Verification items for the finished model (mm, model axes). Give positions to 0.01 mm unless a question says otherwise; leave off trailing zeros. Loops run counter-clockwise (first coordinate to the right, second up) from the corner with the lowest first, then second, coordinate; pieces in that order, holes last. Notation, with made-up numbers: (-32, 10) - (-20, 10) arc R20 cw to (-20, 40) - close; hole circle Ø9 at (82.25, 41.5). An arc over 180 degrees is marked (long way). One line per item, written item: value. Start each with the question number.
1. Gauge pin test, flat ends, axial feed: pin 1 (8 mm diameter, centred on x = -364, y = -24.5, fed in from -Z); pin 2 (10 mm diameter, centred on y = -25.5, z = 73, fed in from -X); pin 3 (3 mm diameter, centred on x = -150.5, y = -46, fed in from +Z). Record the tip position at first contact, or that the pin passes through.
2. Sectioned sample at A-A (x = 0). Record the cut outline in (y, z).
3. Scan lines: L1, parallel to Z at x = 64, y = -24.5; L2, parallel to X at y = -55, z = -211.5; L3, parallel to X at y = -11.5, z = -253. Record each from-to range of solid material in increasing order. Write a range as [from, to].
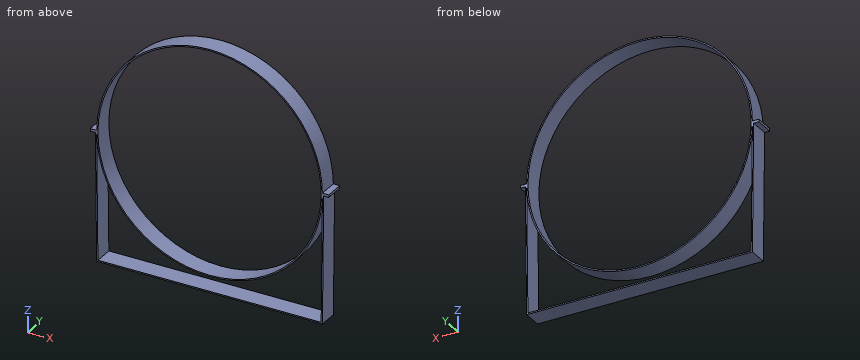
from build123d import *

# Parameters (mm, degrees)
F0_R     = 350
F1_DEPTH = 60


with BuildPart() as f1:
    # F0 (on Front) → F1 (new body)
    with BuildSketch(Plane.XZ):
        with BuildLine():
            ThreePointArc((353.9774, -4), (353.99435, -2.000032), (354, 0))
            ThreePointArc((354, 0), (353.99435, 2.000032), (353.9774, 4))
            ThreePointArc((353.9774, 4), (0, 354), (-353.9774, 4))
            ThreePointArc((-353.9774, 4), (-354, 0), (-353.9774, -4))
            ThreePointArc((-353.9774, -4), (0, -354), (353.9774, -4))
        make_face()
        Circle(F0_R, mode=Mode.SUBTRACT)
        with BuildLine():
            ThreePointArc((353.9774, 4), (353.99435, 2.000032), (354, 0))
            ThreePointArc((354, 0), (353.99435, -2.000032), (353.9774, -4))
            Line((353.9774, -4), (357.9776, -4))
            Line((357.9776, -4), (373.9774, -4))
            Line((373.9774, -4), (373.9774, 0))
            Line((373.9774, 0), (373.9774, 4))
            Line((373.9774, 4), (353.9774, 4))
        make_face()
        Polygon((357.9776, -4), (353.9774, -4), (350.017602, -399.940196), (-350.017602, -399.940196), (-353.9774, -4), (-357.9776, -4), (-353.9774, -403.979997), (353.9774, -403.979997), align=None)
        with BuildLine():
            ThreePointArc((-353.9774, -4), (-354, 0), (-353.9774, 4))
            Line((-353.9774, 4), (-373.9774, 4))
            Line((-373.9774, 4), (-373.9774, 0))
            Line((-373.9774, 0), (-373.9774, -4))
            Line((-373.9774, -4), (-357.9776, -4))
            Line((-357.9776, -4), (-353.9774, -4))
        make_face()
    extrude(amount=F1_DEPTH)


solid = f1.part
Results are:
1. pin 1: stops at z = -4
1. pin 2: stops at x = -347.41
1. pin 3: stops at z = 321.12
2. outline: (-60, -403.98) - (0, -403.98) - (0, -399.94) - (-60, -399.94) - close; (-60, -354) - (0, -354) - (0, -350) - (-60, -350) - close; (-60, 350) - (0, 350) - (0, 354) - (-60, 354) - close
3. L1: z = [-403.98, -399.94], [-348.17, -344.1], [344.1, 348.17]
3. L2: x = [-355.9, -351.9], [-283.87, -278.87], [278.87, 283.87], [351.9, 355.9]
3. L3: x = [-355.49, -351.49], [-247.6, -241.85], [241.85, 247.6], [351.49, 355.49]
